Could you check a few things on this drawing? It's one solid part, dimensions in mm from its lowest x, y, z. Coordinates: 2 decimals unless noted, no trailing zeros. Write each loop counter-clockwise with the first axis right and the second up, starting at its lowest first coordinate (ties: lowest second). Pieces come first, ordered by that corner, then holes. Notation, with made-up numbers: M 24,64.25 L 40,64.25 A22 ccw 40,101.25 Z; hole C 50.25,8.25 d2. An arc over 180 degrees is marked long. Use a Markdown table: item, result.
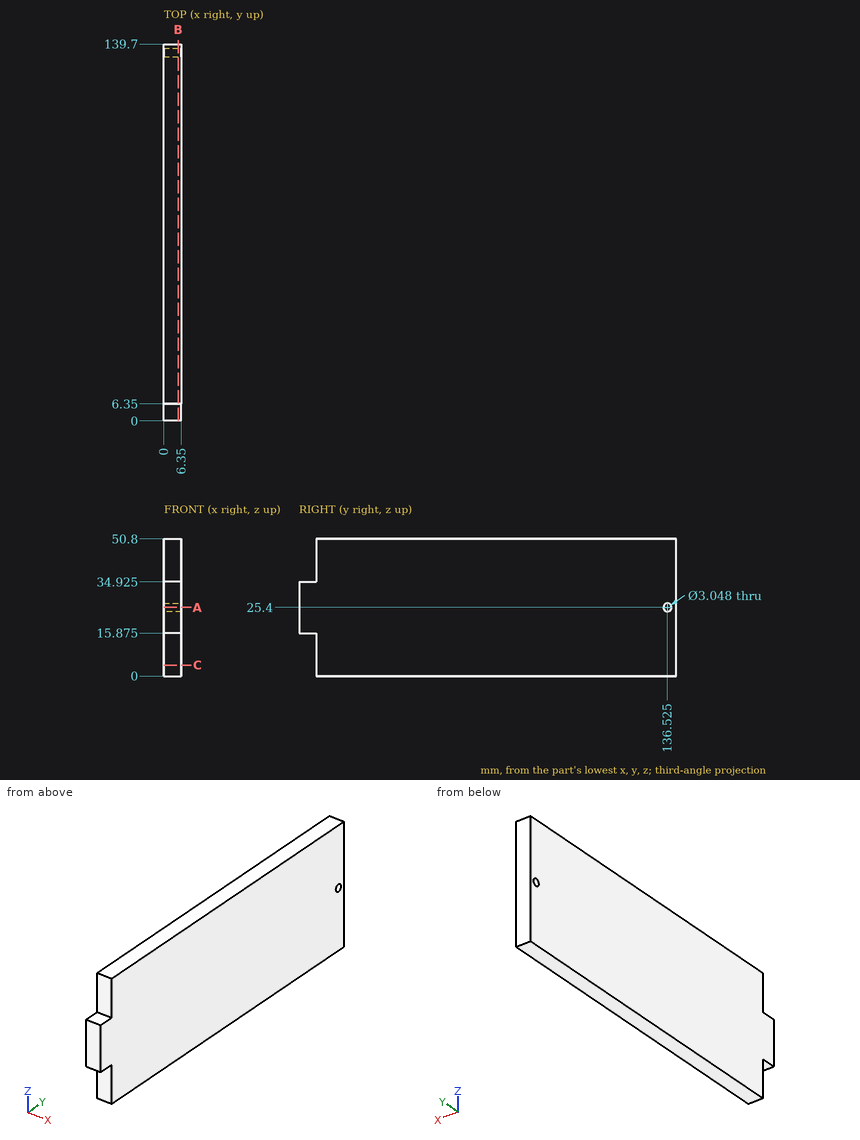
1. Will these pins go through, and if not, where does the flat tip stop? pin 1 Ø1.9 at (x, y) = (4, 4) entering from +Z (3 decimals); pin 2 Ø3 at (x, z) = (4.5, 41.5) entering from -Y.
Answers follow:
| item | result |
|---|---|
| pin 1 | stops at z = 34.925 |
| pin 2 | stops at y = 6.35 |
2. Suppose I cut it at C-C on z = 4. Write out the boundary of the cut face in (x, y).
Answers follow:
| item | result |
|---|---|
| outline | M 0,6.35 L 6.35,6.35 L 6.35,139.7 L 0,139.7 Z |
3. Suppose I cut it at A-A on z = 25.4. Write out the boundary of the cut face in (x, y).
Answers follow:
| item | result |
|---|---|
| outline | M 0,0 L 6.35,0 L 6.35,135 L 0,135 Z; M 0,138.05 L 6.35,138.05 L 6.35,139.7 L 0,139.7 Z |
4. Suppose I cut it at B-B on x = 5.25. Write out the boundary of the cut face in (y, z) (3 decimals).
Answers follow:
| item | result |
|---|---|
| outline | M 0,15.875 L 6.35,15.875 L 6.35,0 L 139.7,0 L 139.7,50.8 L 6.35,50.8 L 6.35,34.925 L 0,34.925 Z; hole C 136.525,25.4 d3.048 |
5. I need wall thicknesses on probe 1 along Y at (x, z) = (2.75, 25.4); probe 2 along Y at (x, z) = (4.75, 11.5). Which ranges of each line are inside material? Lowest first, please.
Answers follow:
| item | result |
|---|---|
| probe 1 | y = 0 to 135, 138.05 to 139.7 |
| probe 2 | y = 6.35 to 139.7 |
